```python
from build123d import *

# Parameters (mm, degrees)
SKETCH2_R           = 5
SKETCH2_R_2         = 1.5
BOSS_EXTRUDE1_DEPTH = 4
FILLET1_R           = 0.5
FILLET2_R           = 0.5


with BuildPart() as part:
    # Sketch2 → Boss-Extrude1 (new body)
    with BuildSketch(Plane(origin=(0, 0, 0), x_dir=(1, 0, 0), z_dir=(0, 1, 0))):
        Circle(SKETCH2_R)
        Circle(SKETCH2_R_2, mode=Mode.SUBTRACT)
    extrude(amount=BOSS_EXTRUDE1_DEPTH)

    # Fillet1
    fillet1_edges = [part.edges().sort_by_distance(p)[0] for p in [
        (-5, 0, 0),
        (-5, 4, 0),
    ]]
    fillet(fillet1_edges, radius=FILLET1_R)

    # Fillet2
    fillet2_edges = [part.edges().sort_by_distance(p)[0] for p in [
        (-1.5, 0, 0),
        (-1.5, 4, 0),
    ]]
    fillet(fillet2_edges, radius=FILLET2_R)


solid = part.part
```
Design review of the part built by this model. Coordinates are the model's own, in mm. Coordinates: 2 decimals unless noted, no trailing zeros. Write each loop counter-clockwise with the first axis right and the second up, starting at its lowest first coordinate (ties: lowest second). Pieces come first, ordered by that corner, then holes.
1) Add section B-B (z = 0). Write out the cut boundary in (x, y).
2) Mouldability with a two-part tool opening along X and no side actions: class faces 1 (the cylindrical face through (-1.5, 1.98, -0.07)), 2 (the flat face through (1, 0, 2)), 3 (the cylindrical face through (-1.08, 1.98, 4.88)) as +X half, -X half, draft (parallel to the pull), parting line (faces both ways), or undercut.
3) Add section C-C (y = 2.9). Write out the cut boundary in (x, z), plus the area to 3 significant figures.
4) Insertion check: pin 1 (1 mm diameter, centred on x = -2, y = 3, fed in from -Z); pin 2 (1.5 mm diameter, centred on y = 2.5, z = -2.5, fed in from -X); pin 3 (5 mm diameter, centred on x = 0, z = 0, fed in from -Y); pin 4 (2 mm diameter, centred on x = 3.5, y = 2, fed in from +Z). Each pin has a flat end and moves straight along its axis. Give the tip position at first contact, or say it passes through.
5) To check wall thickness, follow L1, parallel to Z at x = 0, y = 2.6; L2, parallel to Z at x = -1, y = 0.25. State the ranges of each line that lie inside material, in increasing order.
6) Add section A-A (x = 0). Write out the cut boundary in (y, z), plus the area to 3 significant figures.
Check result:
1. outline: (-5, 0.5) arc R0.5 ccw to (-4.5, 0) - (-2, 0) arc R0.5 ccw to (-1.5, 0.5) - (-1.5, 3.5) arc R0.5 ccw to (-2, 4) - (-4.5, 4) arc R0.5 ccw to (-5, 3.5) - close; (1.5, 0.5) arc R0.5 ccw to (2, 0) - (4.5, 0) arc R0.5 ccw to (5, 0.5) - (5, 3.5) arc R0.5 ccw to (4.5, 4) - (2, 4) arc R0.5 ccw to (1.5, 3.5) - close
2. face 1: undercut
2. face 2: draft
2. face 3: parting line
3. outline: circle Ø10 at (0, 0); hole circle Ø3 at (0, 0)
3. area: 71.5 mm2
4. pin 1: stops at z = -4.77
4. pin 2: stops at x = -4.68
4. pin 3: stops at y = 0
4. pin 4: stops at z = 4.33
5. L1: z = -5 to -1.5, 1.5 to 5
5. L2: z = -4.83 to -1.21, 1.21 to 4.83
6. outline: (0, -4.5) arc R0.5 ccw to (0.5, -5) - (3.5, -5) arc R0.5 ccw to (4, -4.5) - (4, -2) arc R0.5 ccw to (3.5, -1.5) - (0.5, -1.5) arc R0.5 ccw to (0, -2) - close; (0, 2) arc R0.5 ccw to (0.5, 1.5) - (3.5, 1.5) arc R0.5 ccw to (4, 2) - (4, 4.5) arc R0.5 ccw to (3.5, 5) - (0.5, 5) arc R0.5 ccw to (0, 4.5) - close
6. area: 27.6 mm2
